The model under review builds one solid part; all positions refer to its coordinate system, in mm. A direction names the side the tool comes from. Round coordinates to 2 decimals unless told otherwise and drop trailing zeros. Loops run counter-clockwise (first coordinate to the right, second up) from the corner with the lowest first, then second, coordinate; pieces in that order, holes last. Notation, with made-up numbers: (41.25, -27) -> (87.25, -27) arc R19 cw to (87.25, 2) -> close; hole circle Ø1 at (88.25, 89). An arc over 180 degrees is marked (long way). Return JSON: item names as keys, results as strings. Group by question number.
```python
from build123d import *

# Parameters (mm, degrees)
F0_W     = 45.4
F0_H     = 48.2
F0_W_2   = 31.4
F0_H_2   = 34.2
F1_DEPTH = 2
F2_DEPTH = 13
F3_DEPTH = 13
F5_W     = 42.2
F5_H     = 7
F6_DEPTH = 80


with BuildPart() as f1:
    # F0 (on Top) → F1 (new body)
    with BuildSketch(Plane.XY):
        Rectangle(F0_W, F0_H)
        Polygon((-20.7, -22.1), (-20.7, 22.1), (-10.7, 22.1), (-10, 22.1), (-0.35, 22.1), (0.35, 22.1), (10, 22.1), (10.7, 22.1), (20.7, 22.1), (20.7, -22.1), (10.7, -22.1), (10, -22.1), (0.35, -22.1), (-0.35, -22.1), (-10, -22.1), (-10.7, -22.1), align=None, mode=Mode.SUBTRACT)
        with BuildLine():
            Line((-10.7, 22.1), (-20.7, 22.1))
            Line((-20.7, 22.1), (-20.7, -22.1))
            Line((-20.7, -22.1), (-10.7, -22.1))
            ThreePointArc((-10.7, -22.1), (-10.35, -21.75), (-10, -22.1))
            Line((-10, -22.1), (-0.35, -22.1))
            ThreePointArc((-0.35, -22.1), (0, -21.75), (0.35, -22.1))
            Line((0.35, -22.1), (10, -22.1))
            ThreePointArc((10, -22.1), (10.35, -21.75), (10.7, -22.1))
            Line((10.7, -22.1), (20.7, -22.1))
            Line((20.7, -22.1), (20.7, 22.1))
            Line((20.7, 22.1), (10.7, 22.1))
            ThreePointArc((10.7, 22.1), (10.35, 21.75), (10, 22.1))
            Line((10, 22.1), (0.35, 22.1))
            ThreePointArc((0.35, 22.1), (0, 21.75), (-0.35, 22.1))
            Line((-0.35, 22.1), (-10, 22.1))
            ThreePointArc((-10, 22.1), (-10.35, 21.75), (-10.7, 22.1))
        make_face()
        Rectangle(F0_W_2, F0_H_2, mode=Mode.SUBTRACT)
    extrude(amount=F1_DEPTH)

    # F0 (on Top) → F2 (join)
    with BuildSketch(Plane.XY):
        Rectangle(F0_W, F0_H)
        Polygon((-20.7, -22.1), (-20.7, 22.1), (-10.7, 22.1), (-10, 22.1), (-0.35, 22.1), (0.35, 22.1), (10, 22.1), (10.7, 22.1), (20.7, 22.1), (20.7, -22.1), (10.7, -22.1), (10, -22.1), (0.35, -22.1), (-0.35, -22.1), (-10, -22.1), (-10.7, -22.1), align=None, mode=Mode.SUBTRACT)
    extrude(amount=F2_DEPTH)

    # F0 (on Top) → F3 (join)
    with BuildSketch(Plane.XY):
        with BuildLine():
            Line((-10, 22.1), (-10.7, 22.1))
            ThreePointArc((-10.7, 22.1), (-10.35, 21.75), (-10, 22.1))
        make_face()
        with BuildLine():
            Line((0.35, 22.1), (-0.35, 22.1))
            ThreePointArc((-0.35, 22.1), (0, 21.75), (0.35, 22.1))
        make_face()
        with BuildLine():
            Line((10.7, 22.1), (10, 22.1))
            ThreePointArc((10, 22.1), (10.35, 21.75), (10.7, 22.1))
        make_face()
        with BuildLine():
            ThreePointArc((-10, -22.1), (-10.35, -21.75), (-10.7, -22.1))
            Line((-10.7, -22.1), (-10, -22.1))
        make_face()
        with BuildLine():
            ThreePointArc((0.35, -22.1), (0, -21.75), (-0.35, -22.1))
            Line((-0.35, -22.1), (0.35, -22.1))
        make_face()
        with BuildLine():
            ThreePointArc((10.7, -22.1), (10.35, -21.75), (10, -22.1))
            Line((10, -22.1), (10.7, -22.1))
        make_face()
    extrude(amount=F3_DEPTH)

    # F5 (on face) → F6 (cut)
    with BuildSketch(Plane.YZ.offset(22.7)):
        with Locations((0, 6.5)):
            Rectangle(F5_W, F5_H)
    extrude(amount=-F6_DEPTH, mode=Mode.SUBTRACT)


solid = f1.part
```
1. We need section A-A, the plane z = 3.75. Write out the cut boundary in (x, y).
2. We need section C-C, the plane y = 9. Write out the cut boundary in (x, z).
3. Draft analysis for pull direction Y (two halves, no side actions). For faces 5 (the face through (22.7, 0, 11)), 6 (the face through (22, 21.1, 6)), 7 (the face through (15.7, 0, 1)), state which applies: pulls with the +Y half, pulls with the -Y half, needs draft (parallel to the pull), parting line crosses it, or undercut.
4. We need section D-D, the plane y = -19.5. Write out the cut boundary in (x, z), then the cut area to 3 significant figures.
5. For P1, Ø1, axis at x = 14.5, y = 5.5, coming from the -Z side; P2, Ø6, axis at x = 8.5, y = -16.5, coming from the +Z side, all flat-tipped, find the tip position at first contact; note any pin that passes through.
6. Wall thickness on line 1 (X direction, y = 18, z = 12); line 2 (Y direction, x = 8, z = 11); line 3 (Y direction, x = -13.5, z = 0.5): over which ranges is each line inside the solid? List them lowest first.
7. We need section B-B, the plane x = -13. Write out the cut boundary in (y, z).
8. Tool access review of faces 1 (the face through (-22.7, 0, 11)), 2 (the face through (20.7, 0.1, 10.3)), 3 (the face through (0, -17.1, 1)), 4 (the face through (-22, -21.1, 6)): name each direction out of +Z, -Z, +X, -X, +Y, -Y from which nothing blocks a thin tool from reaching the whole face with its end or side.
Check sheet entries:
{
 "1": {"outline": "(-22.7, -24.1) -> (22.7, -24.1) -> (22.7, -21.1) -> (20.7, -21.1) -> (20.7, -22.1) -> (10.7, -22.1) arc R0.35 ccw to (10, -22.1) -> (0.35, -22.1) arc R0.35 ccw to (-0.35, -22.1) -> (-10, -22.1) arc R0.35 ccw to (-10.7, -22.1) -> (-20.7, -22.1) -> (-20.7, -21.1) -> (-22.7, -21.1) -> close; (-22.7, 21.1) -> (-20.7, 21.1) -> (-20.7, 22.1) -> (-10.7, 22.1) arc R0.35 ccw to (-10, 22.1) -> (-0.35, 22.1) arc R0.35 ccw to (0.35, 22.1) -> (10, 22.1) arc R0.35 ccw to (10.7, 22.1) -> (20.7, 22.1) -> (20.7, 21.1) -> (22.7, 21.1) -> (22.7, 24.1) -> (-22.7, 24.1) -> close"},
 "2": {"outline": "(-22.7, 0) -> (-15.7, 0) -> (-15.7, 2) -> (-20.7, 2) -> (-20.7, 3) -> (-22.7, 3) -> close; (-22.7, 10) -> (-20.7, 10) -> (-20.7, 13) -> (-22.7, 13) -> close; (15.7, 0) -> (22.7, 0) -> (22.7, 3) -> (20.7, 3) -> (20.7, 2) -> (15.7, 2) -> close; (20.7, 10) -> (22.7, 10) -> (22.7, 13) -> (20.7, 13) -> close"},
 "3": {"face 5": "needs draft", "face 6": "undercut", "face 7": "undercut"},
 "4": {"outline": "(-22.7, 0) -> (22.7, 0) -> (22.7, 3) -> (20.7, 3) -> (20.7, 2) -> (-20.7, 2) -> (-20.7, 3) -> (-22.7, 3) -> close; (-22.7, 10) -> (-20.7, 10) -> (-20.7, 13) -> (-22.7, 13) -> close; (20.7, 10) -> (22.7, 10) -> (22.7, 13) -> (20.7, 13) -> close", "area": "107 mm²"},
 "5": {"P1": "passes through", "P2": "stops at z = 2"},
 "6": {"line 1": "x = -22.7 to -20.7, 20.7 to 22.7", "line 2": "y = -24.1 to -22.1, 22.1 to 24.1", "line 3": "y = -24.1 to -17.1, 17.1 to 24.1"},
 "7": {"outline": "(-24.1, 0) -> (-17.1, 0) -> (-17.1, 2) -> (-22.1, 2) -> (-22.1, 13) -> (-24.1, 13) -> close; (17.1, 0) -> (24.1, 0) -> (24.1, 13) -> (22.1, 13) -> (22.1, 2) -> (17.1, 2) -> close"},
 "8": {"face 1": "+Z, -Z, -X, +Y, -Y", "face 2": "+Z", "face 3": "+Z, -Z", "face 4": "+X, -X"}
}
